```python
from build123d import *

# Parameters (mm, degrees)
F0_W      = 30
F0_H      = 3
F1_DEPTH  = 25
F2_W      = 30
F2_H      = 3
F3_DEPTH  = 5
F5_D      = 2.15
F5_DEPTH  = 29.55
F5_TIP    = 0.6459251655
F6_W      = 3
F6_H      = 4.4
F7_DEPTH  = 12
F8_W      = 3
F8_H      = 7
F9_DEPTH  = 3
F10_W     = 3
F10_H     = 7
F11_DEPTH = 3


with BuildPart() as f1:
    # F0 (on Top) → F1 (new body, symmetric)
    with BuildSketch(Plane.XY):
        Rectangle(F0_W, F0_H)
    extrude(amount=F1_DEPTH, both=True)

    # F2 (on face) → F3 (join)
    with BuildSketch(Plane.XZ.offset(1.5)):
        with Locations((0, 19.1)):
            Rectangle(F2_W, F2_H)
        with Locations((0, -15.9)):
            Rectangle(F2_W, F2_H)
    extrude(amount=F3_DEPTH)

    # F5
    with Locations(Plane.XZ.offset(1.5)):
        with Locations((0, 23.1)):
            Hole(F5_D / 2, depth=F5_DEPTH)
            with Locations((0, 0, -(F5_DEPTH + F5_TIP / 2))):  # 118° drill point
                Cone(0, F5_D / 2, F5_TIP, mode=Mode.SUBTRACT)

    # F6 (on face) → F7 (join)
    with BuildSketch(Plane.XZ.offset(1.5)):
        with Locations((-8.5, 15.4)):
            Rectangle(F6_W, F6_H)
        with Locations((-2.5, 15.4)):
            Rectangle(F6_W, F6_H)
        with Locations((-8.5, -12.2)):
            Rectangle(F6_W, F6_H)
        with Locations((-2.5, -12.2)):
            Rectangle(F6_W, F6_H)
    extrude(amount=F7_DEPTH)

    # F8 (on face) → F9 (join, through all)
    with BuildSketch(Plane.XY.offset(17.6)):
        with Locations((-8.5, -10)):
            Rectangle(F8_W, F8_H)
        with Locations((-2.5, -10)):
            Rectangle(F8_W, F8_H)
    extrude(amount=F9_DEPTH)

    # F10 (on face) → F11 (join, through all)
    with BuildSketch(Plane(origin=(0, 0, -14.4), x_dir=(1, 0, 0), z_dir=(0, 0, -1))):
        with Locations((-8.5, 10)):
            Rectangle(F10_W, F10_H)
        with Locations((-2.5, 10)):
            Rectangle(F10_W, F10_H)
    extrude(amount=F11_DEPTH)


solid = f1.part
```
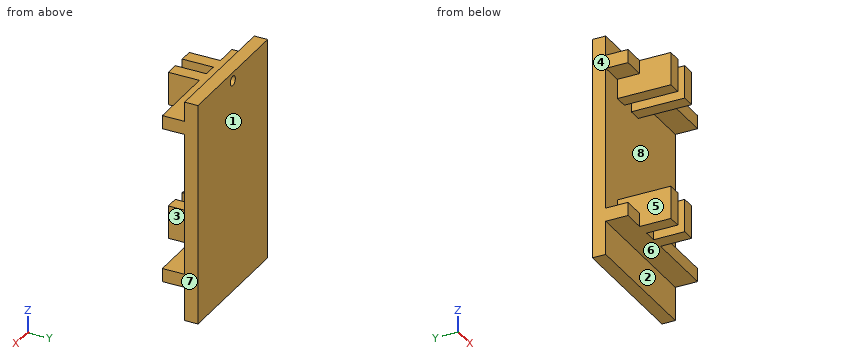
Work out the finished part from the listing and answer in its coordinate system (mm). Face numbers are marked on the shaded views. A direction names the side the tool comes from. Give positions to 0.01 mm unless a question says otherwise; leave off trailing zeros. Order: outer loops, then holes, each group sorted by start corner. A loop starts at its lowest first (then second) coordinate and runs counter-clockwise, first axis right, second up.
1. Section A-A, the plane y = -2 is taken. Determine the outline of the cut face in (x, z), and give its area (3 significant figures).
Result sheet:
outline: (-15, -17.4) - (15, -17.4) - (15, -14.4) - (-1, -14.4) - (-1, -10) - (-4, -10) - (-4, -14.4) - (-7, -14.4) - (-7, -10) - (-10, -10) - (-10, -14.4) - (-15, -14.4) - close; (-15, 17.6) - (-10, 17.6) - (-10, 13.2) - (-7, 13.2) - (-7, 17.6) - (-4, 17.6) - (-4, 13.2) - (-1, 13.2) - (-1, 17.6) - (15, 17.6) - (15, 20.6) - (-15, 20.6) - close
area: 233 mm2
2. Section D-D, the plane z = 23.1 is taken. Determine the outline of the cut face in (x, y) (3 decimals), and give its area (4 significant figures).
Result sheet:
outline: (-15, -1.5) - (-1.075, -1.5) - (-1.075, 1.5) - (-15, 1.5) - close; (1.075, -1.5) - (15, -1.5) - (15, 1.5) - (1.075, 1.5) - close
area: 83.55 mm2
3. Each of these flat-tipped pins is pushed along its axis until it touches: P1, Ø0.9, axis at x = -2.5, y = -5.5, coming from the -Z side; P2, Ø2, axis at y = -10, z = -14.5, coming from the +X side; P3, Ø1.5, axis at x = -5.5, z = -15.5, coming from the -Y side. Where does it stop, or does it pass through?
Result sheet:
P1: stops at z = -17.4
P2: stops at x = -1
P3: stops at y = -6.5
4. The mould has two halves that part along Z. Classify the marked faces 6, 7 and 8: released by +Z, released by -Z, zero draft, split by the parting line, or undercut.
Result sheet:
face 6: released by -Z
face 7: zero draft
face 8: undercut
5. For the marked faces 1, 2, 3, 4 and 5, determine the directions among +Z, -Z, +X, -X, +Y, -Y from which every point of the face is accessible in a straight line to the end or side of a thin tool.
Result sheet:
face 1: +Z, -Z, +X, -X, +Y
face 2: -Z, +X, -X, -Y
face 3: +X, -Y
face 4: +Z, -Z, -X, +Y, -Y
face 5: -X, -Y
6. Section C-C, the plane y = -8 is taken. Determine the outline of the cut face in (x, z).
Result sheet:
outline: (-10, -17.4) - (-7, -17.4) - (-7, -10) - (-10, -10) - close; (-10, 13.2) - (-7, 13.2) - (-7, 20.6) - (-10, 20.6) - close; (-4, -17.4) - (-1, -17.4) - (-1, -10) - (-4, -10) - close; (-4, 13.2) - (-1, 13.2) - (-1, 20.6) - (-4, 20.6) - close
7. Section B-B, the plane x = 0 is taken. Determine the outline of the cut face in (y, z) (3 decimals).
Result sheet:
outline: (-6.5, -17.4) - (-1.5, -17.4) - (-1.5, -25) - (1.5, -25) - (1.5, 22.025) - (-1.5, 22.025) - (-1.5, 20.6) - (-6.5, 20.6) - (-6.5, 17.6) - (-1.5, 17.6) - (-1.5, -14.4) - (-6.5, -14.4) - close; (-1.5, 24.175) - (1.5, 24.175) - (1.5, 25) - (-1.5, 25) - close
8. Straight lines are drawn through the part: L1, parallel to Z at x = -10.75, y = -5; L2, parallel to Z at x = 0, y = 0.45 (3 decimals); L3, parallel to X at y = -5.25, z = 15.5. For each, find the intervals that lie inside material, in ascending order.
Result sheet:
L1: z = -17.4 to -14.4, 17.6 to 20.6
L2: z = -25 to 22.025, 24.175 to 25
L3: x = -10 to -7, -4 to -1
